Design review of the part shown in the three views and the two pictorial views. Dimensions are in mm from the part's minimum x, y and z. A direction names the side the tool comes from. Round coordinates to 2 decimals unless told otherwise and drop trailing zeros. Write each loop counter-clockwise with the first axis right and the second up, starting at its lowest first coordinate (ties: lowest second). Pieces come first, ordered by that corner, then holes. Notation, with made-up numbers: (79, -32) -> (110, -32) arc R31 ccw to (110, -5) -> close; hole circle Ø9 at (83, 1.25). An arc over 180 degrees is marked (long way). Answer as a JSON object with one key per item and string values. Group by question number.
1) Machinability: for the marked faces 4 and 5, which of the approach directions +Z, -Z, +X, -X, +Y, -Y give a long, thin tool a straight path to every point of the face, cutting with its end or side? Answer none if there is none.
2) Mouldability with a two-part tool opening along X and no side actions: class the marked faces 1, 2 and 3 as pulls with the +X half, pulls with the -X half, needs draft (parallel to the pull), parting line crosses it, or undercut.
3) We need section D-D, the plane x = 6. Write out the cut boundary in (y, z).
4) We need section C-C, the plane z = 39. Write out the cut boundary in (x, y), then the cut area to 3 significant figures.
5) To check wall thickness, follow probe 1 along X at (y, z) = (6.6, 21.5); probe 2 along X at (y, z) = (3.55, 21.5) (1 decimal); probe 3 along Y at (x, z) = (35, 19.5). State the ranges of each line that lie inside material, in increasing order. Write a range as [from, to].
6) We need section B-B, the plane x = 21.5. Write out the cut boundary in (y, z) (1 decimal).
7) We need section A-A, the plane z = 21.5. Write out the cut boundary in (x, y) (1 decimal).
8) Insertion check: pin 1 Ø2 at (x, z) = (26.5, 18.5) entering from -Y; pin 2 Ø4 at (y, z) = (3.5, 13.5) entering from -X; pin 3 Ø6.5 at (x, z) = (21.5, 21.5) entering from -Y; pin 4 Ø4.5 at (x, z) = (11.5, 21) entering from +Y. Each pin has a flat end and moves straight along its axis. Give the tip position at first contact, or say it passes through.
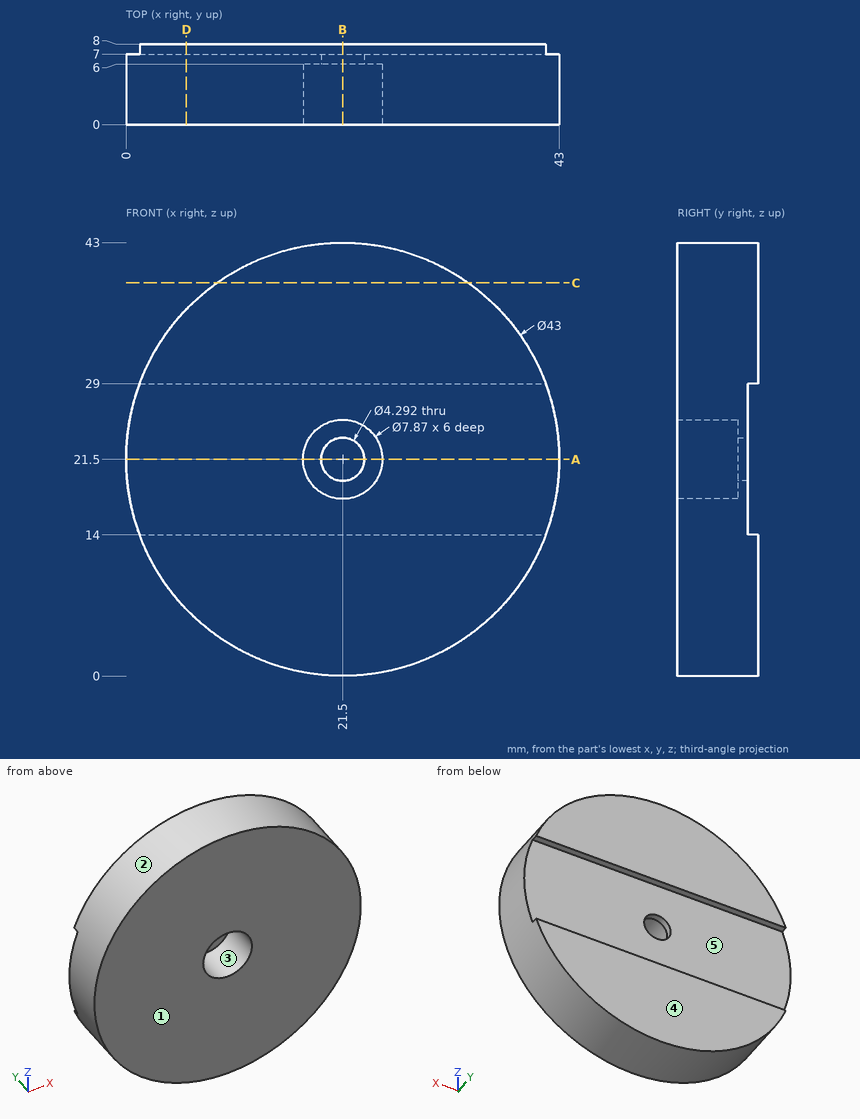
Here are the results:
{
 "1": {"face 4": "+Z, -Z, +X, -X, +Y", "face 5": "+X, -X, +Y"},
 "2": {"face 1": "needs draft", "face 2": "parting line crosses it", "face 3": "undercut"},
 "3": {"outline": "(0, 6.6) -> (8, 6.6) -> (8, 14) -> (7, 14) -> (7, 29) -> (8, 29) -> (8, 36.4) -> (0, 36.4) -> close"},
 "4": {"outline": "(9.01, 0) -> (33.99, 0) -> (33.99, 8) -> (9.01, 8) -> close", "area": "200 mm^2"},
 "5": {"probe 1": "x = [0, 19.35], [23.65, 43]", "probe 2": "x = [0, 17.6], [25.4, 43]", "probe 3": "y = [0, 7]"},
 "6": {"outline": "(0, 0) -> (8, 0) -> (8, 14) -> (7, 14) -> (7, 19.4) -> (6, 19.4) -> (6, 17.6) -> (0, 17.6) -> close; (0, 25.4) -> (6, 25.4) -> (6, 23.6) -> (7, 23.6) -> (7, 29) -> (8, 29) -> (8, 43) -> (0, 43) -> close"},
 "7": {"outline": "(0, 0) -> (17.6, 0) -> (17.6, 6) -> (19.4, 6) -> (19.4, 7) -> (0, 7) -> close; (23.6, 6) -> (25.4, 6) -> (25.4, 0) -> (43, 0) -> (43, 7) -> (23.6, 7) -> close"},
 "8": {"pin 1": "stops at y = 0", "pin 2": "stops at x = 0.85", "pin 3": "stops at y = 6", "pin 4": "stops at y = 7"}
}
